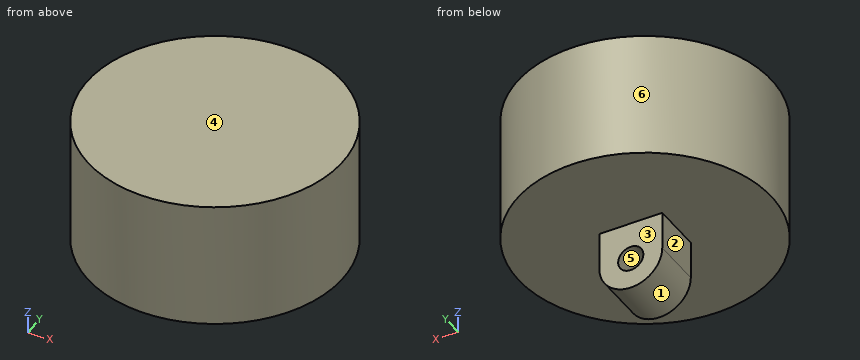
from build123d import *

# Parameters (mm, degrees)
SKETCH1_R           = 5
BOSS_EXTRUDE1_DEPTH = 5
SKETCH2_R           = 0.5
BOSS_EXTRUDE2_DEPTH = 1


with BuildPart() as part:
    # Sketch1 → Boss-Extrude1 (new body)
    with BuildSketch(Plane.XY):
        Circle(SKETCH1_R)
    extrude(amount=BOSS_EXTRUDE1_DEPTH)

    # Sketch2 → Boss-Extrude2 (add, symmetric)
    with BuildSketch(Plane(origin=(0, 0, 0), x_dir=(1, 0, 0), z_dir=(0, 1, 0))):
        with BuildLine():
            Line((-1.25, 0), (1.25, 0))
            Line((1.25, 0), (1.25, 1.5))
            ThreePointArc((1.25, 1.5), (0, 2.75), (-1.25, 1.5))
            Line((-1.25, 1.5), (-1.25, 0))
        make_face()
        with Locations(Location((0, 1.5, 0), (0, 0, 270))):
            Circle(SKETCH2_R, mode=Mode.SUBTRACT)
    extrude(amount=BOSS_EXTRUDE2_DEPTH, both=True)


solid = part.part
Work out the finished part from the listing and answer in its coordinate system (mm). Face numbers are marked on the shaded views. A direction names the side the tool comes from. Coordinates: 2 decimals unless noted, no trailing zeros. Order: outer loops, then holes, each group sorted by start corner. A loop starts at its lowest first (then second) coordinate and runs counter-clockwise, first axis right, second up. Notation, with made-up numbers: (-4.5, 33) - (-0.5, 33) arc R19 cw to (-0.5, 50) - close; hole circle Ø6 at (43.25, 89). An arc over 180 degrees is marked (long way). Put each result on its own line as item: value. Start each with the question number.
1) Find section C-C (z = 4). Give the vertices of the cut face in (x, y), plus the area to 3 significant figures.
2) Find the intervals of material crossed by line 1 (X direction, y = -0.45, z = -1.5); line 2 (Z direction, x = -1, y = -3.25); line 3 (Y direction, x = 3.5, z = 4), in increasing order. Write a range as from..to.
3) For a pull along Z with two mould halves and no side action, classify the marked faces 4, 5 and 6 as released by +Z, released by -Z, zero draft, split by the parting line, or undercut.
4) Find section A-A (x = 0). Give the vertices of the cut face in (y, z), plus the area to 3 significant figures.
5) For the marked faces 1, 2 and 3, determine the directions among +Z, -Z, +X, -X, +Y, -Y from which every point of the face is accessible in a straight line to the end or side of a thin tool.
6) Find section D-D (x = -3). Give the vertices of the cut face in (y, z).
7) Flat-ended cylindrical pins translate along their axes: pin 1 (1.5 mm diameter, centred on y = 1, z = -2, fed in from +X); pin 2 (4 mm diameter, centred on x = 3.5, z = 3, fed in from +Y); pin 3 (4 mm diameter, centred on y = -2.5, z = 1.5, fed in from +X). Find the tip coordinate at first contact, or state that the pin passes through.
8) Find section B-B (y = 0). Give the vertices of the cut face in (x, z).
Results list:
1. outline: circle Ø10 at (0, 0)
1. area: 78.5 mm^2
2. line 1: x = -1.25..-0.5, 0.5..1.25
2. line 2: z = 0..5
2. line 3: y = -3.57..3.57
3. face 4: released by +Z
3. face 5: undercut
3. face 6: zero draft
4. outline: (-5, 0) - (-1, 0) - (-1, -1) - (1, -1) - (1, 0) - (5, 0) - (5, 5) - (-5, 5) - close; (-1, -2.75) - (1, -2.75) - (1, -2) - (-1, -2) - close
4. area: 53.5 mm^2
5. face 1: -Z, +Y, -Y
5. face 2: -Z, -X, +Y, -Y
5. face 3: -Z, +X, -X, +Y
6. outline: (-4, 0) - (4, 0) - (4, 5) - (-4, 5) - close
7. pin 1: stops at x = 1.25
7. pin 2: stops at y = 4.77
7. pin 3: stops at x = 4.97
8. outline: (-5, 0) - (-1.25, 0) - (-1.25, -1.5) arc R1.25 ccw to (1.25, -1.5) - (1.25, 0) - (5, 0) - (5, 5) - (-5, 5) - close; hole circle Ø1 at (0, -1.5)
